from build123d import *

# Parameters (mm, degrees)
F1_DEPTH = 16
F2_R     = 1.49999


# Not quite as in the source:
# - a fillet or chamfer is up to 0.001 mm smaller than in the source, because OpenCascade refuses the exact size


with BuildPart() as f1:
    # F0 (on Front) → F1 (new body)
    with BuildSketch(Plane.XZ):
        with BuildLine():
            ThreePointArc((0, -33), (-26.6113648632, -19.5150008997), (-31.4739884393, 9.9190751445))
            Line((-31.4739884393, 9.9190751445), (-45, -33))
            Line((-45, -33), (0, -33))
        make_face()
        with BuildLine():
            Line((5, -30), (0, -30))
            ThreePointArc((0, -30), (-27.7163859753, -11.480502971), (-21.2132034356, 21.2132034356))
            Line((-21.2132034356, 21.2132034356), (-23.3345237792, 23.3345237792))
            ThreePointArc((-23.3345237792, 23.3345237792), (-28.213238354, 17.1176278024), (-31.4739884393, 9.9190751445))
            ThreePointArc((-31.4739884393, 9.9190751445), (-26.6113648632, -19.5150008997), (0, -33))
            ThreePointArc((0, -33), (2.5072470561, -32.9046153632), (5, -32.6190128606))
            Line((5, -32.6190128606), (5, -30))
        make_face()
        with BuildLine():
            Line((5, -33), (5, -32.6190128606))
            ThreePointArc((5, -32.6190128606), (2.5072470561, -32.9046153632), (0, -33))
            Line((0, -33), (5, -33))
        make_face()
    extrude(amount=F1_DEPTH)

    # F2 (radius 1.5 in the source; OpenCascade refuses exactly that, so slightly less here)
    f2_edges = [f1.edges().sort_by_distance(p)[0] for p in [
        (-21.213203, -8, 21.213203),
        (-23.334524, -8, 23.334524),
        (5, -8, -30),
    ]]
    fillet(f2_edges, radius=F2_R)


solid = f1.part
Check sheet for the modelled part. Datum: model origin and axes. Units: mm. A direction names the side the tool comes from. Give positions to 0.01 mm unless a question says otherwise; leave off trailing zeros. Loops run counter-clockwise (first coordinate to the right, second up) from the corner with the lowest first, then second, coordinate; pieces in that order, holes last. Notation, with made-up numbers: M 38,33 L 73,33 A33 cw 73,69 Z; hole C 2.5,-31.5 d7. An arc over 180 degrees is marked long. Return JSON: item names as keys, results as strings. Group by question number.
1. Cross-section at D-D on x = -6. Record the boundary of the cut face in (y, z).
2. Go/stop test with flat-tipped pins: pin 1 (4 mm diameter, centred on y = -8.5, z = -24.5, fed in from -X); pin 2 (1.1 mm diameter, centred on x = 2.5, y = -8, fed in from +Z); pin 3 (5 mm diameter, centred on y = -3.5, z = 10.5, fed in from +X); pin 4 (4 mm diameter, centred on x = -32, z = -17.5, fed in from +Y). Record where each tip stops, or that it passes through.
3. Tool access check on faces 1 (the cylindrical face through (-21.81, -8.11, 21.21)), 2 (the flat face through (2, -8, -30)). Record the directions out of +Z, -Z, +X, -X, +Y, -Y that give a thin tool (end or side, any length) a straight path to the whole face; none if there is none.
4. Cross-section at C-C on z = -22. Record the boundary of the cut face in (x, y).
5. Thickness scan on L1, parallel to Z at x = -22, y = -11; L2, parallel to X at y = -13, z = -26; L3, parallel to X at y = -5, z = 14.5. Record the ranges inside material, lowest first.
6. Cross-section at A-A on x = -27. Record the boundary of the cut face in (y, z), plus the area to 3 significant figures.
Return value:
{
 "1": {"outline": "M -16,-33 L 0,-33 L 0,-29.39 L -16,-29.39 Z"},
 "2": {"pin 1": "x = -42.95", "pin 2": "z = -30", "pin 3": "x = -27.04", "pin 4": "y = 0"},
 "3": {"face 1": "+X, +Y, -Y", "face 2": "+Z, +X, +Y, -Y"},
 "4": {"outline": "M -41.53,-16 L -20.4,-16 L -20.4,0 L -41.53,0 Z"},
 "5": {"L1": "-33 to -20.4, 20.46 to 21.92", "L2": "-42.79 to -14.97", "L3": "-29.64 to -26.26"},
 "6": {"outline": "M -16,-33 L 0,-33 L 0,-13.08 L -16,-13.08 Z; M -16,13.08 L 0,13.08 L 0,18.97 L -16,18.97 Z", "area": "413 mm^2"}
}
